Autodesk Inventor part; units mm, degrees
ref_plane "YZ Plane" through (0, 0, 0) normal (1, 0, 0) x (0, 1, 0)
ref_plane "XZ Plane" through (0, 0, 0) normal (0, 1, 0) x (-1, 0, 0)
ref_plane "XY Plane" through (0, 0, 0) normal (0, 0, 1) x (1, 0, 0)
sketch "Sketch1" plane through (0, 0, 0) normal (0, 1, 0) x (-1, 0, 0)
  circle A0 centre (0, 0) radius 3.95
  dimension "d0" = 7.9
extrude "Extrusion1" add sketch "Sketch1" along normal blind 160
sketch "Sketch2" plane through (0, 160, 0) normal (0, 1, 0) x (1, 0, 0)
  line L0 (-0.9, -1.9) -> (0.9, -1.9)
  line L1 (0.9, -1.9) -> (0.9, 1.9)
  line L2 (0.9, 1.9) -> (-0.9, 1.9)
  line L3 (-0.9, 1.9) -> (-0.9, -1.9)
  line L4 (-0.9, -1.9) -> (0.9, 1.9) construction
  line L5 (0.9, -1.9) -> (-0.9, 1.9) construction
  point P0 (0, 0)
  dimension "d3" = 3.8
  dimension "d4" = 1.8
extrude "Extrusion2" add sketch "Sketch2" along normal blind 30
sketch "Sketch3" plane through (0.9, 160, 1.9) normal (1, 0, 0) x (0, 0, -1)
  line L0 (0, 30) -> (3.8, 30)
  line L1 (1.9, 30) -> (1.9, 25)
  circle A0 centre (1.9, 25) radius 1.1
  line L2 (1.9, 25) -> (1.9, 15)
  line L3 (3.8, 0) -> (3.8, 30)
  circle A1 centre (1.9, 15) radius 1.1
  point P0 (1.9, -160)
  dimension "d7" = 5
  dimension "d8" = 2.2
  dimension "d9" = 10
  dimension "d10" = 2.2
hole "Hole1" at (0.9, 185, 0) at (0.9, 175, 0) direction (-1, 0, 0) diameter 2 end through all
properties part number "Stereotax adaptor v4"
The model under review builds one solid part; all positions refer to its coordinate system, in mm. A direction names the side the tool comes from. Round coordinates to 2 decimals unless told otherwise and drop trailing zeros. Order: outer loops, then holes, each group sorted by start corner. A loop starts at its lowest first (then second) coordinate and runs counter-clockwise, first axis right, second up.
(1) Tool access review of faces 1 (the face through (-0.9, 174.8, -1.3)), 2 (the face through (0.9, 174.8, 1.3)), 3 (the face through (3.135, 78.88, 2.404)): name each direction out of +Z, -Z, +X, -X, +Y, -Y from which nothing blocks a thin tool from reaching the whole face with its end or side.
Working result:
face 1: +Z, -Z, -X, +Y
face 2: +Z, -Z, +X, +Y
face 3: +Y, -Y
(2) Take a section at A-A, the plane y = 168.5. State the section outline as (x, z) points.
Working result:
outline: (-0.9, -1.9) - (0.9, -1.9) - (0.9, 1.9) - (-0.9, 1.9) - close
(3) Wall thickness on L1, parallel to Y at x = 0.5, z = 0; L2, parallel to Z at x = 0.5, y = 175; L3, parallel to Y at x = 2.25, z = -0.75: over which ranges is each line inside the solid? List them lowest first.
Working result:
L1: y = 0 to 174, 176 to 184, 186 to 190
L2: z = -1.9 to -1, 1 to 1.9
L3: y = 0 to 160
(4) Take a section at B-B, the plane y = 130. State the section outline as (x, z) points.
Working result:
outline: circle Ø7.9 at (0, 0)
(5) For P1, Ø3, axis at y = 170, z = -0.5, coming from the -X side; P2, Ø2.5, axis at y = 175, z = 0, coming from the +X side; P3, Ø1.4, axis at x = 0.5, y = 173, coming from the -Z side, all flat-tipped, find the tip position at first contact; note any pin that passes through.
Working result:
P1: stops at x = -0.9
P2: stops at x = 0.9
P3: stops at z = -1.9
